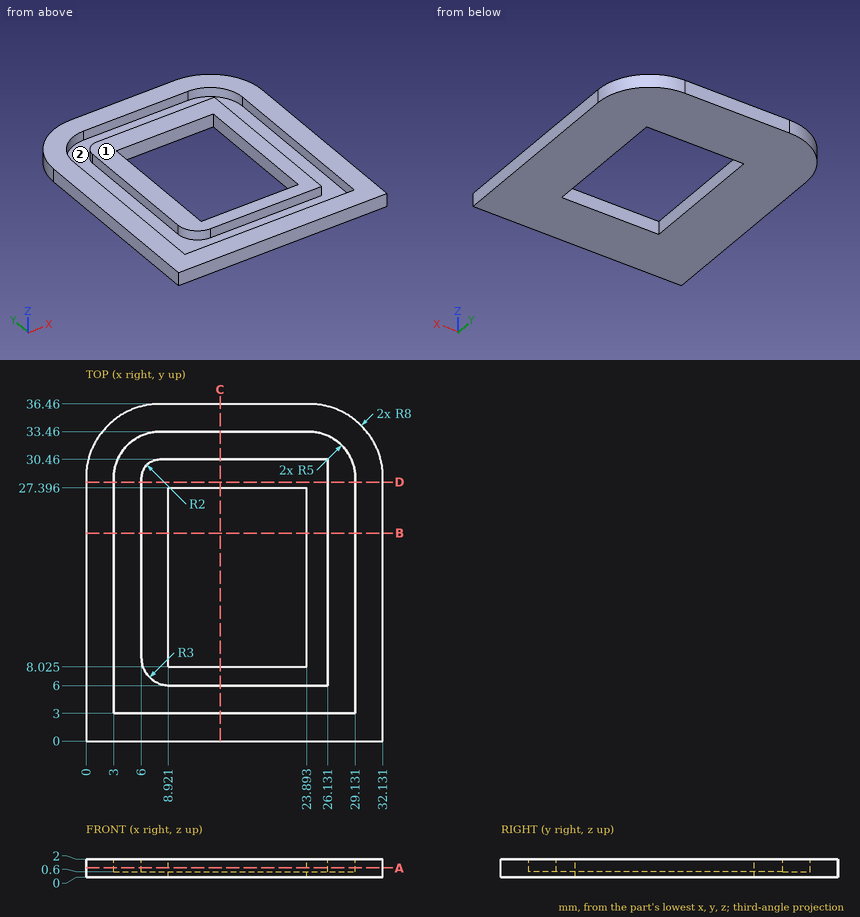
Check sheet for the drawn part. Datum: minimum x, y, z corner. Units: mm. Round coordinates to 2 decimals unless told otherwise and drop trailing zeros. Order: outer loops, then holes, each group sorted by start corner. A loop starts at its lowest first (then second) coordinate and runs counter-clockwise, first axis right, second up. Notation, with made-up numbers: (10, 29) -> (63, 29) arc R32 ccw to (63, 62) -> close; hole circle Ø10 at (27.25, 75). An arc over 180 degrees is marked (long way). Put each result on its own line as item: value.
1) Section check B-B (y = 22.5). Record the cut outline in (x, z).
Final values:
outline: (0, 0) -> (8.92, 0) -> (8.92, 2) -> (6, 2) -> (6, 0.6) -> (3, 0.6) -> (3, 2) -> (0, 2) -> close; (23.89, 0) -> (32.13, 0) -> (32.13, 2) -> (29.13, 2) -> (29.13, 0.6) -> (26.13, 0.6) -> (26.13, 2) -> (23.89, 2) -> close
2) Section check C-C (x = 14.5). Record the cut outline in (y, z) (1 decimal).
Final values:
outline: (0, 0) -> (8, 0) -> (8, 2) -> (6, 2) -> (6, 0.6) -> (3, 0.6) -> (3, 2) -> (0, 2) -> close; (27.4, 0) -> (36.5, 0) -> (36.5, 2) -> (33.5, 2) -> (33.5, 0.6) -> (30.5, 0.6) -> (30.5, 2) -> (27.4, 2) -> close
3) Section check D-D (y = 28). Record the cut outline in (x, z).
Final values:
outline: (0, 0) -> (32.13, 0) -> (32.13, 2) -> (29.13, 2) -> (29.13, 0.6) -> (26.13, 0.6) -> (26.13, 2) -> (6, 2) -> (6, 0.6) -> (3, 0.6) -> (3, 2) -> (0, 2) -> close
4) Section check A-A (z = 1.05). Record the cut outline in (x, y) (1 decimal).
Final values:
outline: (0, 0) -> (32.1, 0) -> (32.1, 28.5) arc R8 ccw to (24.1, 36.5) -> (8, 36.5) arc R8 ccw to (0, 28.5) -> close; (6, 9) arc R3 ccw to (9, 6) -> (26.1, 6) -> (26.1, 30.5) -> (8, 30.5) arc R2 ccw to (6, 28.5) -> close; hole (3, 3) -> (29.1, 3) -> (29.1, 28.5) arc R5 ccw to (24.1, 33.5) -> (8, 33.5) arc R5 ccw to (3, 28.5) -> close; hole (8.9, 8) -> (23.9, 8) -> (23.9, 27.4) -> (8.9, 27.4) -> close
5) Material ranges on line 1 (X direction, y = 25, z = 0.75); line 2 (Y direction, x = 10.5, z = 1.65) (1 decimal); line 3 (X direction, y = 27.5, z = 1.05), recorded low to high.
Final values:
line 1: x = 0 to 3, 6 to 8.92, 23.89 to 26.13, 29.13 to 32.13
line 2: y = 0 to 3, 6 to 8, 27.4 to 30.5, 33.5 to 36.5
line 3: x = 0 to 3, 6 to 26.13, 29.13 to 32.13
6) Depth check by flat-ended pin: pin 1 (1 mm diameter, centred on x = 15, z = 1, fed in from -Y). Enter the tip coordinate at first touch or a pass-through.
Final values:
pin 1: stops at y = 0
7) Mould release check, pull along Y, two halves, no side actions. Record for the marked faces 1 and 2: +Y half, -Y half, draft (parallel to the pull), parting line (faces both ways), or undercut.
Final values:
face 1: draft
face 2: undercut
